```python
from build123d import *

# Parameters (mm, degrees)
SKETCH1_R           = 3
BOSS_EXTRUDE1_DEPTH = 3
FILLET1_R           = 3
FILLET2_R           = 3
FILLET3_R           = 3


with BuildPart() as part:
    # Sketch1 → Boss-Extrude1 (new body)
    with BuildSketch(Plane.XY):
        with BuildLine():
            Line((27.478538516, 6), (0, 6))
            ThreePointArc((0, 6), (-6, 0), (0, -6))
            Line((0, -6), (30.017, -6))
            ThreePointArc((30.017, -6), (34.259640687, -4.242640687), (36.017, 0))
            Line((36.017, 0), (36.017, 11.821966509))
            Line((36.017, 11.821966509), (62.002996518, 26.812896598))
            Line((62.002996518, 26.812896598), (76.138457922, 19.6799669))
            Line((76.138457922, 19.6799669), (82.48746868, 23.342615602))
            Line((82.48746868, 23.342615602), (79.078019732, 29.252717774))
            Line((79.078019732, 29.252717774), (63.506652751, 36.784076585))
            Line((63.506652751, 36.784076585), (27.478538516, 16))
            Line((27.478538516, 16), (27.478538516, 6))
        make_face()
        Circle(SKETCH1_R, mode=Mode.SUBTRACT)
        with Locations((30.017, 0)):
            Circle(SKETCH1_R, mode=Mode.SUBTRACT)
    extrude(amount=BOSS_EXTRUDE1_DEPTH)

    # Fillet1
    fillet1_edges = [part.edges().sort_by_distance(p)[0] for p in [
        (27.478538516, 16, 1.5),
    ]]
    fillet(fillet1_edges, radius=FILLET1_R)

    # Fillet2
    fillet2_edges = [part.edges().sort_by_distance(p)[0] for p in [
        (27.478538516, 6, 1.5),
    ]]
    fillet(fillet2_edges, radius=FILLET2_R)

    # Fillet3
    fillet3_edges = [part.edges().sort_by_distance(p)[0] for p in [
        (63.506652751, 36.784076585, 1.5),
        (62.002996518, 26.812896598, 1.5),
        (36.017, 11.821966509, 1.5),
    ]]
    fillet(fillet3_edges, radius=FILLET3_R)


solid = part.part
```
Could you check a few things on this model? Use its own coordinates, in mm. A direction names the side the tool comes from. Coordinates: 2 decimals unless noted, no trailing zeros. Loops run counter-clockwise (first coordinate to the right, second up) from the corner with the lowest first, then second, coordinate; pieces in that order, holes last.
1) Please list where these lines run through material, in increasing order: line 1 along X through (y, z) = (-1.5, 1.15); line 2 along Y through (x, z) = (8, 1.8); line 3 along X through (y, z) = (22, 2.25).
Reported:
line 1: x = -5.81 to -2.6, 2.6 to 27.42, 32.62 to 35.83
line 2: y = -6 to 6
line 3: x = 37.88 to 53.66, 71.54 to 80.16
2) Imagine slicing it at C-C (x = 17). List the corners of the cut face in (y, z) for me.
Reported:
outline: (-6, 0) - (6, 0) - (6, 3) - (-6, 3) - close
3) Thinking about a two-plate mould opening in X: for faces 4 (the face through (63.5, 36.39, 1.52)), 5 (the face through (26.62, 6.9, 1.52)), 6 (the face through (79.269, 21.486, 1.479)), 7 (the face through (48.897, 19.252, 1.479)), which applies, released by +X, released by -X, zero draft, split by the parting line, or undercut?
Reported:
face 4: split by the parting line
face 5: released by -X
face 6: released by +X
face 7: undercut
4) Will these pins go through, and if not, where does the flat tip stop? pin 1 Ø1.5 at (x, z) = (34.5, 1) entering from +Y; pin 2 Ø0.9 at (y, z) = (6, 2) entering from +X.
Reported:
pin 1: stops at y = 20.48
pin 2: stops at x = 36.02
5) Imagine slicing it at A-A (z = 0.6). List the corners of the cut face in (x, y) for me, and give its area (3 significant figures).
Reported:
outline: (0, -6) - (30.02, -6) arc R6 ccw to (36.02, 0) - (36.02, 10.09) arc R3 cw to (37.52, 12.69) - (60.6, 26) arc R3 cw to (63.45, 26.08) - (76.14, 19.68) - (82.49, 23.34) - (79.08, 29.25) - (64.94, 36.09) arc R3 ccw to (62.13, 35.99) - (28.98, 16.87) arc R3 ccw to (27.48, 14.27) - (27.48, 9) arc R3 cw to (24.48, 6) - (0, 6) arc R6 ccw to start; hole circle Ø6 at (0, 0); hole circle Ø6 at (30.02, 0)
area: 963 mm2
6) Imagine slicing it at D-D (y = 32). List the corners of the cut face in (x, z) for me, and give its area (3 significant figures).
Reported:
outline: (55.21, 0) - (73.4, 0) - (73.4, 3) - (55.21, 3) - close
area: 54.6 mm2
7) Which directions (+Z, -Z, +X, -X, +Y, -Y) give clear straight access to the entire face, cutting with the end or side of a thin tool? Please do faces 1 (the face through (72.106, 32.625, 1.479)), 2 (the face through (12, 6, 1)), 3 (the face through (36.017, 5, 1)).
Reported:
face 1: +Z, -Z, +X, +Y
face 2: +Z, -Z, -X, +Y
face 3: +Z, -Z, +X, -Y
8) Imagine slicing it at B-B (x = 31.5). List the corners of the cut face in (y, z) for me.
Reported:
outline: (-5.81, 0) - (-2.61, 0) - (-2.61, 3) - (-5.81, 3) - close; (2.61, 0) - (18.32, 0) - (18.32, 3) - (2.61, 3) - close
